Design review of the part built by this model. Coordinates are the model's own, in mm. A direction names the side the tool comes from. Give positions to 0.01 mm unless a question says otherwise; leave off trailing zeros. Order: outer loops, then holes, each group sorted by start corner. A loop starts at its lowest first (then second) coordinate and runs counter-clockwise, first axis right, second up. Notation, with made-up numbers: (-40, -4) -> (-34, -4) arc R16 ccw to (-34, 18) -> close; hole circle Ø2 at (72, -34). An arc over 180 degrees is marked (long way). Use a Markdown table: item, result. Add a question column.
```python
from build123d import *

# Parameters (mm, degrees)
SKETCH_R        = 39
SKETCH_R_2      = 30
PAD006_DEPTH    = 10
SKETCH008_R     = 37.5
SKETCH008_R_2   = 31.5
POCKET002_DEPTH = 0.5
SKETCH009_R     = 37.5
SKETCH009_R_2   = 31.5
POCKET003_DEPTH = 0.5


with BuildPart() as part:
    # Sketch → Pad006 (new body)
    with BuildSketch(Plane.XY):
        Circle(SKETCH_R)
        Circle(SKETCH_R_2, mode=Mode.SUBTRACT)
    extrude(amount=PAD006_DEPTH)

    # Sketch008 → Pocket002 (cut)
    with BuildSketch(Plane.XY.offset(10)):
        Circle(SKETCH008_R)
        Circle(SKETCH008_R_2, mode=Mode.SUBTRACT)
    extrude(amount=-POCKET002_DEPTH, mode=Mode.SUBTRACT)

    # Sketch009 → Pocket003 (cut)
    with BuildSketch(Plane.XY):
        Circle(SKETCH009_R)
        Circle(SKETCH009_R_2, mode=Mode.SUBTRACT)
    extrude(amount=POCKET003_DEPTH, mode=Mode.SUBTRACT)


solid = part.part
```
1) For L1, parallel to Y at x = 0, z = 0.25; L2, parallel to Y at x = 0.5, z = 6; L3, parallel to Z at x = 33, y = -5, list the stretches that pass through material, from the lowest coordinate up. Write a range as [from, to].
2) The part is to be moulded in two halves that separate along X. For faces 1 (the cylindrical face through (-5.077, 38.668, 4.93)), 2 (the cylindrical face through (-4.88, 37.18, 9.75)), 3 (the flat face through (-20, 32, 0)), say which applies: +X half, -X half, draft (parallel to the pull), parting line (faces both ways), or undercut.
3) Machinability: for faces 4 (the flat face through (28, -12, 0)), 5 (the flat face through (-9, 31, 9.5)), 6 (the cylindrical face through (-4.101, 31.232, 0.246)), which of the approach directions +Z, -Z, +X, -X, +Y, -Y give a long, thin tool a straight path to every point of the face, cutting with its end or side? Answer none if there is none.
4) Add section A-A (y = 0). Give the boundary of the cut face in (x, z), then the cut area to 3 significant figures.
5) Insertion check: pin 1 (22.5 mm diameter, centred on x = -7, y = 16.5, fed in from -Z); pin 2 (2 mm diameter, centred on x = -28.5, z = 1.5, fed in from +Y); pin 3 (1.5 mm diameter, centred on x = -23.5, z = 2, fed in from +Y); pin 4 (6 mm diameter, centred on y = -8, z = 3, fed in from +X). Each pin has a flat end and moves straight along its axis. Give the tip position at first contact, or say it passes through.
6) Add section C-C (z = 8.5). Give the boundary of the cut face in (x, y).
Worked answers:
| question | item | result |
|---|---|---|
| 1 | L1 | [-39, -37.5], [-31.5, -30], [30, 31.5], [37.5, 39] |
| 1 | L2 | [-39, -30], [30, 39] |
| 1 | L3 | [0.5, 9.5] |
| 2 | face 1 | parting line |
| 2 | face 2 | undercut |
| 2 | face 3 | draft |
| 3 | face 4 | -Z, +X, -X, +Y, -Y |
| 3 | face 5 | +Z |
| 3 | face 6 | -Z |
| 4 | outline | (-39, 0) -> (-37.5, 0) -> (-37.5, 0.5) -> (-31.5, 0.5) -> (-31.5, 0) -> (-30, 0) -> (-30, 10) -> (-31.5, 10) -> (-31.5, 9.5) -> (-37.5, 9.5) -> (-37.5, 10) -> (-39, 10) -> close; (30, 0) -> (31.5, 0) -> (31.5, 0.5) -> (37.5, 0.5) -> (37.5, 0) -> (39, 0) -> (39, 10) -> (37.5, 10) -> (37.5, 9.5) -> (31.5, 9.5) -> (31.5, 10) -> (30, 10) -> close |
| 4 | area | 168 mm^2 |
| 5 | pin 1 | through |
| 5 | pin 2 | y = 27.65 |
| 5 | pin 3 | y = 31.68 |
| 5 | pin 4 | x = 38.68 |
| 6 | outline | circle Ø78 at (0, 0); hole circle Ø60 at (0, 0) |
